Source: CAD feature listing. Evaluate the final solid. Frame: model axes, mm. Give positions to 0.01 mm unless a question says otherwise; leave off trailing zeros. Loops run counter-clockwise (first coordinate to the right, second up) from the corner with the lowest first, then second, coordinate; pieces in that order, holes last. Notation, with made-up numbers: (34, 72) -> (58, 72) arc R7 ccw to (58, 78) -> close; hole circle Ø8 at (15.25, 26.5). An arc over 180 degrees is marked (long way). Return JSON: item names as keys, results as strings. Group by question number.
(1) Cut plane A-A on x = 111.5. Return loops of the section in (y, z), then the cut area to 3 significant figures.
(2) Ray query, line 1 (X direction, y = -12, z = 0.25) (3 decimals); line 2 (X direction, y = -131, z = 2.3); line 3 (X direction, y = -243, z = 4.1). Return the intervals inside material, ascending. Write a range as from..to.
(3) Cut plane B-B on z = 0.9. Give the number of separate pieces and of enclosed holes in the cut face, then the cut area to 3 significant figures.
(4) Draft query along Z for faces 1 (the face through (124, -140, 0)), 2 (the face through (124, -140, 5.08)). Return one class per face: released by +Z, released by -Z, zero draft, split by the parting line, or undercut.
```python
from build123d import *

# Parameters (mm, degrees)
F0_W     = 251.524948
F0_H     = 283.958055
F0_R     = 1.7272
F0_W_2   = 9.525
F0_H_2   = 9.525
F1_DEPTH = 5.08


with BuildPart() as f1:
    # F0 (on Top) → F1 (new body)
    with BuildSketch(Plane.XY):
        with Locations((125.762474, -141.979028)):
            Rectangle(F0_W, F0_H)
        with Locations((4.7625, -279.195555)):
            Circle(F0_R, mode=Mode.SUBTRACT)
        with Locations((60.325, -279.195555)):
            Circle(F0_R, mode=Mode.SUBTRACT)
        with Locations((92.9275, -269.670555)):
            Rectangle(F0_W_2, F0_H_2, mode=Mode.SUBTRACT)
        with Locations((100.870474, -243.82244)):
            Circle(F0_R, mode=Mode.SUBTRACT)
        with Locations((100.870474, -234.04344)):
            Circle(F0_R, mode=Mode.SUBTRACT)
        with BuildLine():
            Line((105.442474, -229.15394), (146.082474, -229.15394))
            Line((146.082474, -229.15394), (146.082474, -237.91694))
            Line((146.082474, -237.91694), (149.511474, -237.91694))
            ThreePointArc((149.511474, -237.91694), (150.527474, -238.93294), (149.511474, -239.94894))
            Line((149.511474, -239.94894), (146.082474, -239.94894))
            Line((146.082474, -239.94894), (146.082474, -248.71194))
            Line((146.082474, -248.71194), (105.442474, -248.71194))
            Line((105.442474, -248.71194), (105.442474, -239.94894))
            Line((105.442474, -239.94894), (102.013474, -239.94894))
            ThreePointArc((102.013474, -239.94894), (100.997474, -238.93294), (102.013474, -237.91694))
            Line((102.013474, -237.91694), (105.442474, -237.91694))
            Line((105.442474, -237.91694), (105.442474, -229.15394))
        make_face(mode=Mode.SUBTRACT)
        with Locations((95.982059, -173.528755)):
            Circle(F0_R, mode=Mode.SUBTRACT)
        with Locations((134.362469, -269.670555)):
            Rectangle(F0_W_2, F0_H_2, mode=Mode.SUBTRACT)
        with Locations((167.197443, -269.670555)):
            Rectangle(F0_W_2, F0_H_2, mode=Mode.SUBTRACT)
        with Locations((150.654474, -243.82244)):
            Circle(F0_R, mode=Mode.SUBTRACT)
        with Locations((150.654474, -234.04344)):
            Circle(F0_R, mode=Mode.SUBTRACT)
        with Locations((191.199948, -279.195555)):
            Circle(F0_R, mode=Mode.SUBTRACT)
        with Locations((246.762448, -279.195555)):
            Circle(F0_R, mode=Mode.SUBTRACT)
        with Locations((155.542889, -173.528755)):
            Circle(F0_R, mode=Mode.SUBTRACT)
        with Locations((53.866193, -131.412889)):
            Circle(F0_R, mode=Mode.SUBTRACT)
        with Locations((53.866193, -71.852059)):
            Circle(F0_R, mode=Mode.SUBTRACT)
        with Locations((4.7625, -4.7625)):
            Circle(F0_R, mode=Mode.SUBTRACT)
        with Locations((60.325, -4.7625)):
            Circle(F0_R, mode=Mode.SUBTRACT)
        with Locations((92.9275, -14.2875)):
            Rectangle(F0_W_2, F0_H_2, mode=Mode.SUBTRACT)
        with Locations((92.9275, -4.7625)):
            Circle(F0_R, mode=Mode.SUBTRACT)
        with Locations((95.982059, -29.736193)):
            Circle(F0_R, mode=Mode.SUBTRACT)
        with Locations((197.658755, -131.412889)):
            Circle(F0_R, mode=Mode.SUBTRACT)
        with Locations((197.658755, -71.852059)):
            Circle(F0_R, mode=Mode.SUBTRACT)
        with Locations((155.542889, -29.736193)):
            Circle(F0_R, mode=Mode.SUBTRACT)
        with Locations((134.362469, -14.2875)):
            Rectangle(F0_W_2, F0_H_2, mode=Mode.SUBTRACT)
        with Locations((134.362469, -4.7625)):
            Circle(F0_R, mode=Mode.SUBTRACT)
        with Locations((167.197443, -14.2875)):
            Rectangle(F0_W_2, F0_H_2, mode=Mode.SUBTRACT)
        with Locations((167.197443, -4.7625)):
            Circle(F0_R, mode=Mode.SUBTRACT)
        with Locations((191.199948, -4.7625)):
            Circle(F0_R, mode=Mode.SUBTRACT)
        with Locations((246.762448, -4.7625)):
            Circle(F0_R, mode=Mode.SUBTRACT)
    extrude(amount=F1_DEPTH)


solid = f1.part
```
Answers:
{
 "1": {"outline": "(-283.96, 0) -> (-248.71, 0) -> (-248.71, 5.08) -> (-283.96, 5.08) -> close; (-229.15, 0) -> (0, 0) -> (0, 5.08) -> (-229.15, 5.08) -> close", "area": "1,340 mm²"},
 "2": {"line 1": "0..88.165, 97.69..129.6, 139.125..162.435, 171.96..251.525", "line 2": "0..52.19, 55.54..195.98, 199.34..251.52", "line 3": "0..99.35, 102.39..105.44, 146.08..149.14, 152.17..251.52"},
 "3": {"separate pieces": "1", "enclosed holes": "30", "area": "69,900 mm²"},
 "4": {"face 1": "released by -Z", "face 2": "released by +Z"}
}
